from build123d import *

# Parameters (mm, degrees)
F0_W     = 100
F0_H     = 724
F0_R     = 7
F1_DEPTH = 10


with BuildPart() as f1:
    # F0 (on Right) → F1 (new body)
    with BuildSketch(Plane.YZ):
        Rectangle(F0_W, F0_H)
        with Locations((0, -312)):
            Circle(F0_R, mode=Mode.SUBTRACT)
        with Locations((0, 200)):
            Circle(F0_R, mode=Mode.SUBTRACT)
        with Locations((0, 312)):
            Circle(F0_R, mode=Mode.SUBTRACT)
    extrude(amount=F1_DEPTH)


solid = f1.part
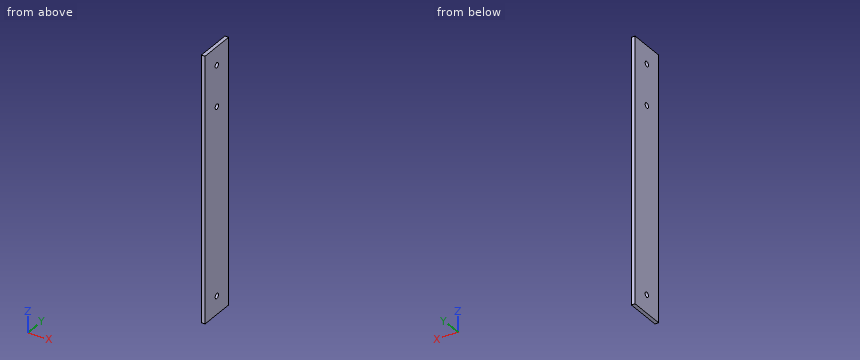
The model under review builds one solid part; all positions refer to its coordinate system, in mm. Round coordinates to 2 decimals unless told otherwise and drop trailing zeros. Order: outer loops, then holes, each group sorted by start corner. A loop starts at its lowest first (then second) coordinate and runs counter-clockwise, first axis right, second up. Notation, with made-up numbers: (15, 74.25) -> (63, 74.25) arc R21 cw to (63, 89.25) -> close; hole circle Ø10 at (42, -1.75). An arc over 180 degrees is marked (long way). Return JSON: item names as keys, results as strings.
1. Take a section at A-A (z = -312). Write out the cut boundary in (x, y).
Answer block:
{"outline": "(0, -50) -> (10, -50) -> (10, -7) -> (0, -7) -> close; (0, 7) -> (10, 7) -> (10, 50) -> (0, 50) -> close"}
2. Take a section at B-B (y = 0). Write out the cut boundary in (x, z), then the cut area to 3 significant figures.
Answer block:
{"outline": "(0, -362) -> (10, -362) -> (10, -319) -> (0, -319) -> close; (0, -305) -> (10, -305) -> (10, 193) -> (0, 193) -> close; (0, 207) -> (10, 207) -> (10, 305) -> (0, 305) -> close; (0, 319) -> (10, 319) -> (10, 362) -> (0, 362) -> close", "area": "6,820 mm²"}
3. For L1, parallel to Z at x = 4, y = 0; L2, parallel to Y at x = 5.75, z = -312, list the stretches that pass through material, from the lowest coordinate up. Write a range as [from, to].
Answer block:
{"L1": "z = [-362, -319], [-305, 193], [207, 305], [319, 362]", "L2": "y = [-50, -7], [7, 50]"}
4. Insertion check: P1, Ø3, axis at y = 27, z = -194.5, coming from the -X side; P2, Ø11, axis at y = 0, z = 200, coming from the -X side. Each pin has a flat end and moves straight along its axis. Give the tip position at first contact, or say it passes through.
Answer block:
{"P1": "stops at x = 0", "P2": "passes through"}
